Design review of the part built by this model. Coordinates are the model's own, in mm. Round coordinates to 2 decimals unless told otherwise and drop trailing zeros. Write each loop counter-clockwise with the first axis right and the second up, starting at its lowest first coordinate (ties: lowest second). Pieces come first, ordered by that corner, then holes. Notation, with made-up numbers: M 70,3.25 L 101,3.25 A25 cw 101,24.25 Z; hole C 79,-36 d6. An arc over 180 degrees is marked long. Use CSV: the item, a comma, the result in double quotes.
from build123d import *

# Parameters (mm, degrees)
SKETCH1_R           = 1.5
SKETCH1_R_2         = 1.672925925
BOSS_EXTRUDE1_DEPTH = 3
SKETCH2_R           = 12.5
CUT_EXTRUDE1_DEPTH  = 4
SKETCH3_R           = 1.5
BOSS_EXTRUDE2_DEPTH = 3


with BuildPart() as part:
    # Sketch1 → Boss-Extrude1 (new body)
    with BuildSketch(Plane(origin=(0, 0, 0), x_dir=(1, 0, 0), z_dir=(0, 1, 0))):
        with BuildLine():
            Line((-16, -21), (16, -21))
            ThreePointArc((16, -21), (19.535533906, -19.535533906), (21, -16))
            Line((21, -16), (21, 16))
            ThreePointArc((21, 16), (19.535533906, 19.535533906), (16, 21))
            Line((16, 21), (-16, 21))
            ThreePointArc((-16, 21), (-19.535533906, 19.535533906), (-21, 16))
            Line((-21, 16), (-21, -16))
            ThreePointArc((-21, -16), (-19.535533906, -19.535533906), (-16, -21))
        make_face()
        with Locations((15.5, 15.5)):
            Circle(SKETCH1_R, mode=Mode.SUBTRACT)
        with Locations((15.5, -15.5)):
            Circle(SKETCH1_R, mode=Mode.SUBTRACT)
        with Locations((-15.5, 15.5)):
            Circle(SKETCH1_R, mode=Mode.SUBTRACT)
        with Locations((-15.5, -15.5)):
            Circle(SKETCH1_R_2, mode=Mode.SUBTRACT)
    extrude(amount=BOSS_EXTRUDE1_DEPTH)

    # Sketch2 → Cut-Extrude1 (cut, through all)
    with BuildSketch(Plane(origin=(0, 3, 0), x_dir=(1, 0, 0), z_dir=(0, 1, 0))):
        Circle(SKETCH2_R)
    extrude(amount=-CUT_EXTRUDE1_DEPTH, mode=Mode.SUBTRACT)

    # Sketch3 → Boss-Extrude2 (add)
    with BuildSketch(Plane(origin=(0, 3, 0), x_dir=(1, 0, 0), z_dir=(0, 1, 0))):
        with BuildLine():
            Line((-24.75, 4.5), (-21, 4.5))
            Line((-21, 4.5), (-21, -4.5))
            Line((-21, -4.5), (-24.75, -4.5))
            ThreePointArc((-24.75, -4.5), (-29.25, 0), (-24.75, 4.5))
        make_face()
        with Locations((-24.75, 0)):
            Circle(SKETCH3_R, mode=Mode.SUBTRACT)
        with BuildLine():
            Line((24.75, -4.5), (21, -4.5))
            Line((21, -4.5), (21, 4.5))
            Line((21, 4.5), (24.75, 4.5))
            ThreePointArc((24.75, 4.5), (29.25, 0), (24.75, -4.5))
        make_face()
        with Locations((24.75, 0)):
            Circle(SKETCH3_R, mode=Mode.SUBTRACT)
    extrude(amount=-BOSS_EXTRUDE2_DEPTH)


solid = part.part
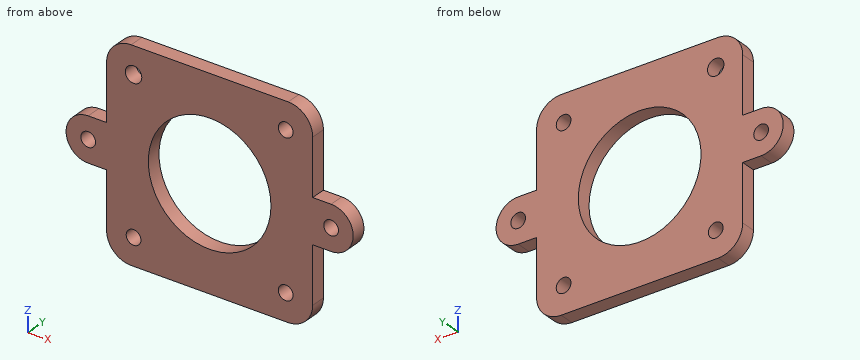
1) Add section D-D on z = -10.5. Write out the cut boundary in (x, y), then the cut area to 3 significant figures.
Answers:
outline,"M -21,0 L -6.78,0 L -6.78,3 L -21,3 Z; M 6.78,0 L 21,0 L 21,3 L 6.78,3 Z"
area,"85.3 mm²"
2) Add section C-C on y = 2.05. Write out the cut boundary in (x, z).
Answers:
outline,"M -24.75,-4.5 L -21,-4.5 L -21,-16 A5 ccw -16,-21 L 16,-21 A5 ccw 21,-16 L 21,-4.5 L 24.75,-4.5 A4.5 ccw 24.75,4.5 L 21,4.5 L 21,16 A5 ccw 16,21 L -16,21 A5 ccw -21,16 L -21,4.5 L -24.75,4.5 A4.5 ccw Z; hole C -24.75,0 d3; hole C -15.5,15.5 d3.35; hole C -15.5,-15.5 d3; hole C 0,0 d25; hole C 15.5,-15.5 d3; hole C 15.5,15.5 d3; hole C 24.75,0 d3"
3) Add section B-B on x = 0. Write out the cut boundary in (y, z).
Answers:
outline,"M 0,-21 L 3,-21 L 3,-12.5 L 0,-12.5 Z; M 0,12.5 L 3,12.5 L 3,21 L 0,21 Z"
4) For pin 1 Ø0.9 at (x, y) = (-23.5, 1.5) entering from -Z; pin 2 Ø1.5 at (x, y) = (22.5, 1.5) entering from +Z; pin 3 Ø2 at (x, z) = (13.5, -2.5) entering from -Y; pin 4 Ø1.8 at (x, z) = (15.5, 15.5) entering from -Y, all flat-tipped, find the tip position at first contact; note any pin that passes through.
Answers:
pin 1,"z = -4.5"
pin 2,"z = 4.5"
pin 3,"y = 0"
pin 4,"through"
5) Wall thickness on line 1 along Z through (x, y) = (-15.5, 2.1); line 2 along X through (y, z) = (0.85, 0); line 3 along X through (y, z) = (1.35, -15.5): over which ranges is each line inside the solid? List them lowest first. Write a range as [from, to].
Answers:
line 1,"[-21, -17], [-14, 13.83], [17.17, 21]"
line 2,"[-29.25, -26.25], [-23.25, -12.5], [12.5, 23.25], [26.25, 29.25]"
line 3,"[-21, -17], [-14, 14], [17, 21]"
6) Add section A-A on z = 0. Write out the cut boundary in (x, y), then the cut area to 3 significant figures.
Answers:
outline,"M -29.25,0 L -26.25,0 L -26.25,3 L -29.25,3 Z; M -23.25,0 L -12.5,0 L -12.5,3 L -23.25,3 Z; M 12.5,0 L 23.25,0 L 23.25,3 L 12.5,3 Z; M 26.25,0 L 29.25,0 L 29.25,3 L 26.25,3 Z"
area,"82.5 mm²"
